Work out the finished part from the listing and answer in its coordinate system (mm). Face numbers are marked on the shaded views. A direction names the side the tool comes from. Give positions to 0.01 mm unless a question says otherwise; leave off trailing zeros. Order: outer loops, then holes, each group sorted by start corner. A loop starts at its lowest first (then second) coordinate and runs counter-clockwise, first axis right, second up. Notation, with made-up numbers: (15.5, 16.5) -> (21.5, 16.5) arc R17 cw to (21.5, 45.5) -> close; hole circle Ø5 at (52, 11). An arc over 180 degrees is marked (long way). Use a Markdown table: item, result. Add a question column.
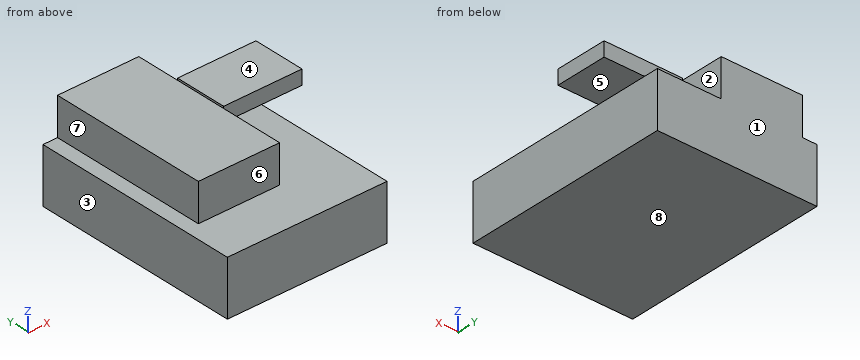
```python
from build123d import *

# Parameters (mm, degrees)
SKIZZE1_W                       = 55
SKIZZE1_H                       = 72
AUFSATZ_LINEAR_AUSTRAGEN1_DEPTH = 19
SKIZZE2_W                       = 28
SKIZZE2_H                       = 55
AUFSATZ_LINEAR_AUSTRAGEN2_DEPTH = 13
SKIZZE3_W                       = 27
SKIZZE3_H                       = 18
AUFSATZ_LINEAR_AUSTRAGEN3_DEPTH = 5


with BuildPart() as part:
    # Skizze1 → Aufsatz-Linear austragen1 (new body)
    with BuildSketch(Plane.XY):
        with Locations((0.254783725, -15.710963455)):
            Rectangle(SKIZZE1_W, SKIZZE1_H)
    extrude(amount=AUFSATZ_LINEAR_AUSTRAGEN1_DEPTH)

    # Skizze2 → Aufsatz-Linear austragen2 (add)
    with BuildSketch(Plane.XY.offset(19)):
        with Locations((-8.245216275, -7.210963455)):
            Rectangle(SKIZZE2_W, SKIZZE2_H)
    extrude(amount=AUFSATZ_LINEAR_AUSTRAGEN2_DEPTH)

    # Skizze3 → Aufsatz-Linear austragen3 (add)
    with BuildSketch(Plane.XY.offset(19)):
        with Locations((28.20593288, 6.289036545)):
            Rectangle(SKIZZE3_W, SKIZZE3_H)
    extrude(amount=AUFSATZ_LINEAR_AUSTRAGEN3_DEPTH)


solid = part.part
```
1) Flat-ended cylindrical pins translate along their axes: pin 1 (5.5 mm diameter, centred on x = 32.5, z = 20.5, fed in from +Y); pin 2 (4 mm diameter, centred on y = -36.5, z = 24, fed in from -X); pin 3 (2.5 mm diameter, centred on x = 25, z = 22.5, fed in from -Y). Find the tip coordinate at first contact, or state that the pin passes through.
2) Which of the six approach directions +Z, -Z, +X, -X, +Y, -Y give full straight-line access (tool end or side, diameter ignored) to the marked faces 4, 5, 6, 7 and 8?
3) The part is cut by section D-D, the plane z = 12. Determine the outline of the cut face in (x, y), then the cut area to 3 significant figures.
4) Straight lines are drawn through the part: line 1 (Z direction, x = 11.5, y = -14.5); line 2 (Y direction, x = -14.5, z = 30); line 3 (Y direction, x = 28.5, z = 21). For each, find the intervals that lie inside material, in ascending order.
5) The part is cut by section B-B, the plane y = -8. Determine the outline of the cut face in (x, z), then the cut area to 3 significant figures.
6) Determine the mould class of the marked faces 1, 2 and 3 for opening direction X: released by +X, released by -X, zero draft, split by the parting line, or undercut.
7) The part is cut by section A-A, the plane z = 22. Determine the outline of the cut face in (x, y), then the cut area to 3 significant figures.
8) The part is cut by section C-C, the plane x = 20. Determine the outline of the cut face in (y, z).
A:
| question | item | result |
|---|---|---|
| 1 | pin 1 | y = 15.29 |
| 1 | pin 2 | x = -22.25 |
| 1 | pin 3 | y = -2.71 |
| 2 | face 4 | +Z, +X, +Y, -Y |
| 2 | face 5 | -Z, +X, +Y, -Y |
| 2 | face 6 | +Z, +X, -X, -Y |
| 2 | face 7 | +Z, -X, +Y, -Y |
| 2 | face 8 | -Z, +X, -X, +Y, -Y |
| 3 | outline | (-27.25, -51.71) -> (27.75, -51.71) -> (27.75, 20.29) -> (-27.25, 20.29) -> close |
| 3 | area | 3,960 mm^2 |
| 4 | line 1 | 0 to 19 |
| 4 | line 2 | -34.71 to 20.29 |
| 4 | line 3 | -2.71 to 15.29 |
| 5 | outline | (-27.25, 0) -> (27.75, 0) -> (27.75, 19) -> (5.75, 19) -> (5.75, 32) -> (-22.25, 32) -> (-22.25, 19) -> (-27.25, 19) -> close |
| 5 | area | 1,410 mm^2 |
| 6 | face 1 | zero draft |
| 6 | face 2 | undercut |
| 6 | face 3 | released by -X |
| 7 | outline | (-22.25, -34.71) -> (5.75, -34.71) -> (5.75, 20.29) -> (-22.25, 20.29) -> close; (14.71, -2.71) -> (41.71, -2.71) -> (41.71, 15.29) -> (14.71, 15.29) -> close |
| 7 | area | 2,030 mm^2 |
| 8 | outline | (-51.71, 0) -> (20.29, 0) -> (20.29, 19) -> (15.29, 19) -> (15.29, 24) -> (-2.71, 24) -> (-2.71, 19) -> (-51.71, 19) -> close |
